```python
from build123d import *

# Parameters (mm, degrees)
ESBO_O1_R                = 2
RESSALTO_EXTRUS_O1_DEPTH = 5
ESBO_O2_R                = 7.750187391
ESBO_O2_R_2              = 4
CORTE_EXTRUS_O1_DEPTH    = 1
CORTE_EXTRUS_O1_TAPER    = 45


with BuildPart() as part:
    # Esboço1 → Ressalto-extrusão1 (new body)
    with BuildSketch(Plane.XY):
        Polygon((2.309401077, -4), (4.618802154, 0), (2.309401077, 4), (-2.309401077, 4), (-4.618802154, 0), (-2.309401077, -4), align=None)
        Circle(ESBO_O1_R, mode=Mode.SUBTRACT)
    extrude(amount=RESSALTO_EXTRUS_O1_DEPTH)

    # Esboço2 → Corte-extrusão1 (cut)
    with BuildSketch(Plane.XY.offset(5)):
        Circle(ESBO_O2_R)
        Circle(ESBO_O2_R_2, mode=Mode.SUBTRACT)
    extrude(amount=-CORTE_EXTRUS_O1_DEPTH, taper=CORTE_EXTRUS_O1_TAPER, mode=Mode.SUBTRACT)


solid = part.part
```
Input: part model. Units: mm. Frame: model coordinates. Give positions to 0.01 mm unless a question says otherwise; leave off trailing zeros. Order: outer loops, then holes, each group sorted by start corner. A loop starts at its lowest first (then second) coordinate and runs counter-clockwise, first axis right, second up. Notation, with made-up numbers: (14, 51) - (52, 51) arc R9 ccw to (52, 64) - close; hole circle Ø8 at (-24, 88.5). An arc over 180 degrees is marked (long way). One line per item, written item: value.
1. Cut plane A-A, the plane z = 1.5. Output: boundary loops of the cut face in (x, y).
Determined:
outline: (-4.62, 0) - (-2.31, -4) - (2.31, -4) - (4.62, 0) - (2.31, 4) - (-2.31, 4) - close; hole circle Ø4 at (0, 0)
2. Draft query along X for faces 1 (the face through (-2, -1, 5)), 2 (the face through (0, -2, 2)), 3 (the face through (4.2, 0, 4.8)). Return one class per face: released by +X, released by -X, zero draft, split by the parting line, or undercut.
Determined:
face 1: zero draft
face 2: undercut
face 3: released by +X
3. Line query: probe 1 along Y at (x, z) = (0, 1.7); probe 2 along X at (y, z) = (1, 4.15); probe 3 along Y at (x, z) = (-1.5, 1.5). Output: solid intervals per line, ascending.
Determined:
probe 1: -4 to -2, 2 to 4
probe 2: -4.04 to -1.73, 1.73 to 4.04
probe 3: -4 to -1.32, 1.32 to 4
4. Pin query (flat end, axial travel): pin 1 Ø3 at (x, y) = (0, 0) entering from +Z (1 decimal); pin 2 Ø2 at (y, z) = (3, 2.5) entering from -X; pin 3 Ø1.5 at (x, z) = (-3.5, 0.5) entering from -Y. Return the tip coordinate at first contact, or that it passes through.
Determined:
pin 1: through
pin 2: x = -3.46
pin 3: y = -3.24
